The listing builds one solid part. Answer for the finished solid, in the listing's coordinates (mm). A direction names the side the tool comes from. Round coordinates to 2 decimals unless told otherwise and drop trailing zeros. Loops run counter-clockwise (first coordinate to the right, second up) from the corner with the lowest first, then second, coordinate; pieces in that order, holes last. Notation, with made-up numbers: M 76,32.25 L 120,32.25 A11 cw 120,53.25 Z; hole C 75,-37 d4. An arc over 180 degrees is marked long. Put each result on its own line as item: value. Start each with the question number.
(1) Section D-D, the plane y = 11 is taken. Determine the outline of the cut face in (x, z), then the cut area to 3 significant figures.
(2) Flat-ended cylindrical pins translate along their axes: P1, Ø2.5, axis at x = -4.5, z = 46, coming from the -Y side; P2, Ø6, axis at y = -13.5, z = 111.5, coming from the +X side; P3, Ø12, axis at y = -12.5, z = 148, coming from the +X side. Find the tip coordinate at first contact, or state that the pin passes through.
(3) Straight lines are drawn through the part: line 1 (X direction, y = -24.5, z = 30); line 2 (Z direction, x = 0, y = -32); line 3 (Z direction, x = 32.5, y = -44). For each, find the intervals that lie inside material, in ascending order.
(4) Determine the mould class of faces 1 (the face through (50, -12, 30)), 2 (the face through (12.1, -25.35, 48.97)), 3 (the face through (-23, -50, 30)) for opening direction X: released by +X, released by -X, zero draft, split by the parting line, or undercut.
(5) Section B-B, the plane x = 0 is taken. Determine the outline of the cut face in (y, z), then the cut area to 3 significant figures.
(6) Section A-A, the plane y = -20 is taken. Determine the outline of the cut face in (x, z).
(7) Section C-C, the plane z = 37 is taken. Determine the outline of the cut face in (x, y).
(8) Which of the six approach directions +Z, -Z, +X, -X, +Y, -Y give full straight-line access (tool end or side, diameter ignored) to faces 4 (the face through (0, 0, 47)), 5 (the face through (-50, -12, 30)), 6 (the face through (-16, -32, 134))?
```python
from build123d import *

# Parameters (mm, degrees)
F0_W     = 100
F0_H     = 100
F1_DEPTH = 60
F2_R     = 20
F3_DEPTH = 150
F5_DEPTH = 100
F6_R     = 22.5
F7_DEPTH = 50


with BuildPart() as f1:
    # F0 (on Top) → F1 (new body)
    with BuildSketch(Plane.XY):
        Rectangle(F0_W, F0_H)
    extrude(amount=F1_DEPTH)

    # F2 (on face) → F3 (join)
    with BuildSketch(Plane.XY.offset(60)):
        with Locations((0, -20)):
            Circle(F2_R)
    extrude(amount=F3_DEPTH)

    # F4 (on face) → F5 (cut)
    with BuildSketch(Plane(origin=(-50, 0, 0), x_dir=(0, -1, 0), z_dir=(-1, 0, 0))):
        Polygon((-23.094011, 30), (11.547005, 10), (11.547005, 50), align=None)
    extrude(amount=-F5_DEPTH, mode=Mode.SUBTRACT)

    # F6 (on face) → F7 (cut)
    with BuildSketch(Plane.XZ.offset(50)):
        with Locations((0, 30)):
            Circle(F6_R)
    extrude(amount=-F7_DEPTH, mode=Mode.SUBTRACT)


solid = f1.part
```
Recorded:
1. outline: M -50,0 L 50,0 L 50,23.02 L -50,23.02 Z; M -50,36.98 L 50,36.98 L 50,60 L -50,60 Z
1. area: 4,600 mm²
2. P1: stops at y = 0
2. P2: stops at x = 19.69
2. P3: stops at x = 19.94
3. line 1: x = -50 to -22.5, 22.5 to 50
3. line 2: z = 0 to 7.5, 52.5 to 210
3. line 3: z = 0 to 60
4. face 1: released by +X
4. face 2: undercut
4. face 3: zero draft
5. outline: M -50,0 L 50,0 L 50,60 L 0,60 L 0,210 L -40,210 L -40,60 L -50,60 L -50,52.5 L 0,52.5 L 0,43.33 L 23.09,30 L 0,16.67 L 0,7.5 L -50,7.5 Z
5. area: 9,440 mm²
6. outline: M -50,0 L 50,0 L 50,60 L 20,60 L 20,210 L -20,210 L -20,60 L -50,60 Z; hole C 0,30 d45
7. outline: M -50,-50 L -21.38,-50 L -21.38,-11.55 L -50,-11.55 Z; M -50,10.97 L 50,10.97 L 50,50 L -50,50 Z; M 21.38,-50 L 50,-50 L 50,-11.55 L 21.38,-11.55 Z
8. face 4: -Y
8. face 5: +Z, -Z, -X, +Y, -Y
8. face 6: +Z
